Answer from the drawing. Dimensions are ordinates in mm from the lowest x, y and z of the part. Coordinates: 2 decimals unless noted, no trailing zeros. Order: outer loops, then holes, each group sorted by start corner. A loop starts at its lowest first (then second) coordinate and runs counter-clockwise, first axis right, second up. Notation, with made-up numbers: (-1.5, 34.25) - (3.5, 34.25) arc R8 cw to (3.5, 38.25) - close; hole circle Ø1 at (50, 49.5). An arc over 180 degrees is marked (long way). Answer as a JSON object with one key per item and string values. Group by question number.
1) Section C-C (x = 1) is taken. Give the vertices of the cut face in (y, z), plus the area to 3 significant figures.
2) Each of these flat-tipped pins is pushed along its axis until it touches: P1, Ø1, axis at y = 6.5, z = 0.5, coming from the +X side; P2, Ø4, axis at x = 3.5, y = 4.04, coming from the +Z side. Where does it stop, or does it pass through?
3) Section A-A (z = 0.95) is taken. Give the vertices of the cut face in (x, y).
4) Find the intervals of material crossed by line 1 along Y through (x, z) = (4.5, 0.45) (1 decimal); line 2 along X through (y, z) = (4.75, 0.2); line 3 along X through (y, z) = (2.5, 0.15) (1 decimal), in increasing order.
5) The mould has two halves that part along X. Classify the marked faces 1, 2 and 3: released by +X, released by -X, zero draft, split by the parting line, or undercut.
6) Section B-B (y = 1) is taken. Give the vertices of the cut face in (x, z).
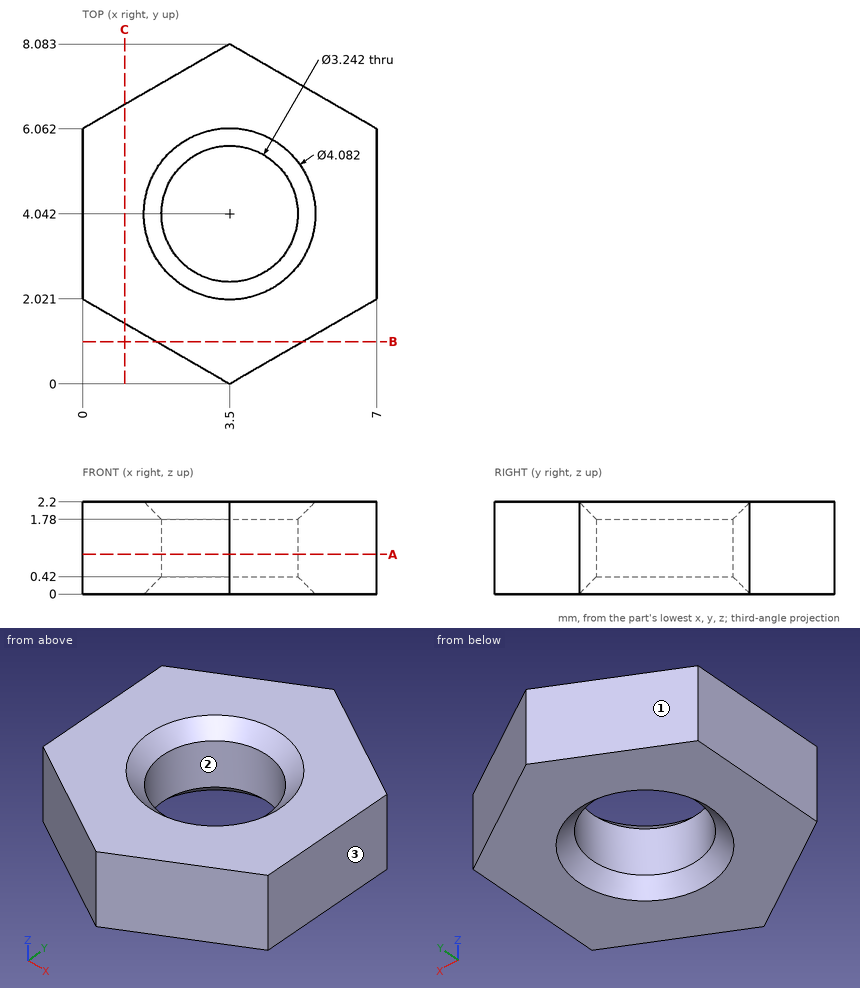
Report:
{
 "1": {"outline": "(1.44, 0) - (6.64, 0) - (6.64, 2.2) - (1.44, 2.2) - close", "area": "11.4 mm²"},
 "2": {"P1": "stops at x = 7", "P2": "stops at z = 2.16"},
 "3": {"outline": "(0, 2.02) - (3.5, 0) - (7, 2.02) - (7, 6.06) - (3.5, 8.08) - (0, 6.06) - close; hole circle Ø3.24 at (3.5, 4.04)"},
 "4": {"line 1": "y = 0.6 to 2.8, 5.3 to 7.5", "line 2": "x = 0 to 1.8, 5.2 to 7", "line 3": "x = 0 to 2.4, 4.6 to 7"},
 "5": {"face 1": "released by -X", "face 2": "undercut", "face 3": "released by +X"},
 "6": {"outline": "(1.77, 0) - (5.23, 0) - (5.23, 2.2) - (1.77, 2.2) - close"}
}
